Input: dimensioned drawing with shaded views. Units: mm. Origin: part minimum x, y, z. A direction names the side the tool comes from. Round coordinates to 2 decimals unless told otherwise and drop trailing zeros. Order: outer loops, then holes, each group sorted by start corner. A loop starts at its lowest first (then second) coordinate and runs counter-clockwise, first axis right, second up.
Item 1: Cut plane D-D on x = 44. Output: boundary loops of the cut face in (y, z), then the cut area to 3 significant figures.
Item 2: Reachability of the marked faces 1, 2 and 3 from +Z, -Z, +X, -X, +Y, -Y: full face, straight path, thin tool, end or side. Return the list, or none.
Item 3: Mould query, pull axis Z, two halves, no side actions, for the marked faces 4, 5 and 6. Classes: released by +Z, released by -Z, zero draft, split by the parting line, or undercut.
Item 4: Cut plane C-C on y = 25.4. Output: boundary loops of the cut face in (x, z), then the cut area to 3 significant figures.
Item 5: First-contact query: pin 1 (2 mm diameter, centred on y = 34.5, z = 56, fed in from +X); pin 2 (3 mm diameter, centred on x = 28.5, z = 29, fed in from +Y); pin 3 (6.5 mm diameter, centred on x = 56.5, z = 36.5, fed in from +Y); pin 4 (4 mm diameter, centred on x = 58.5, z = 37, fed in from -Y). Flat tips, straight axial feed; report the tip coordinate or a pass-through.
Item 6: Cut plane A-A on x = 25.4. Output: boundary loops of the cut face in (y, z).
Item 7: Cut plane B-B on z = 38.1. Output: boundary loops of the cut face in (x, y).
Item 8: Line query: L1, parallel to Z at x = 25.4, y = 25; L2, parallel to X at y = 26, z = 38.1; L3, parallel to X at y = 12, z = 38. Output: solid intervals per line, ascending.
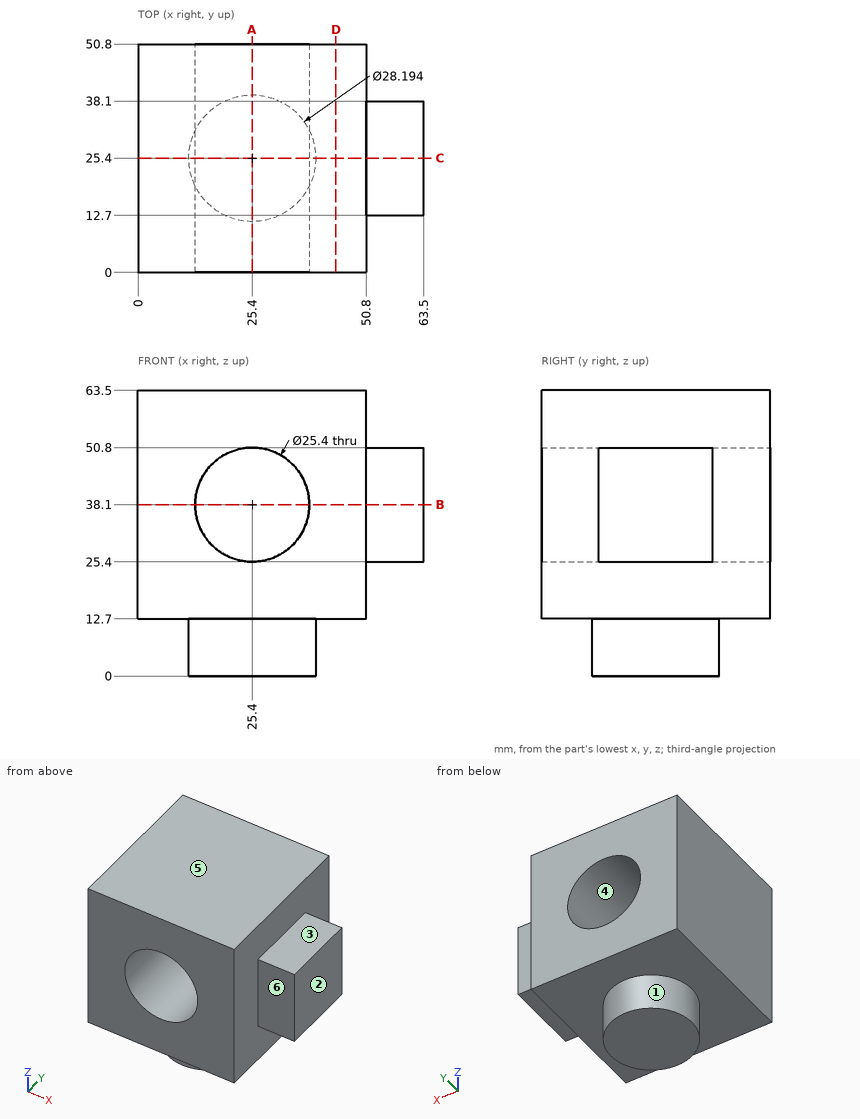
From the geometry:
1. outline: (0, 12.7) - (50.8, 12.7) - (50.8, 63.5) - (0, 63.5) - close
1. area: 2,580 mm2
2. face 1: -Z
2. face 2: +Z, -Z, +X, +Y, -Y
2. face 3: +Z, +X, +Y, -Y
3. face 4: undercut
3. face 5: released by +Z
3. face 6: zero draft
4. outline: (0, 12.7) - (11.3, 12.7) - (11.3, 0) - (39.5, 0) - (39.5, 12.7) - (50.8, 12.7) - (50.8, 25.4) - (63.5, 25.4) - (63.5, 50.8) - (50.8, 50.8) - (50.8, 63.5) - (0, 63.5) - close; hole circle Ø25.4 at (25.4, 38.1)
4. area: 2,750 mm2
5. pin 1: stops at x = 50.8
5. pin 2: passes through
5. pin 3: stops at y = 38.1
5. pin 4: stops at y = 12.7
6. outline: (0, 12.7) - (11.3, 12.7) - (11.3, 0) - (39.5, 0) - (39.5, 12.7) - (50.8, 12.7) - (50.8, 25.4) - (0, 25.4) - close; (0, 50.8) - (50.8, 50.8) - (50.8, 63.5) - (0, 63.5) - close
7. outline: (0, 0) - (12.7, 0) - (12.7, 50.8) - (0, 50.8) - close; (38.1, 0) - (50.8, 0) - (50.8, 12.7) - (63.5, 12.7) - (63.5, 38.1) - (50.8, 38.1) - (50.8, 50.8) - (38.1, 50.8) - close
8. L1: z = 0 to 25.4, 50.8 to 63.5
8. L2: x = 0 to 12.7, 38.1 to 63.5
8. L3: x = 0 to 12.7, 38.1 to 50.8
